from build123d import *

# Parameters (mm, degrees)
F0_R     = 25.4
F0_R_2   = 2.2225
F1_DEPTH = 6.35
F3_R     = 2.54
F2_R     = 2.54
F4_DEPTH = 25.4
F2_R_2   = 7.9375
F5_DEPTH = 25.4
F6_R     = 2.54
F7_DEPTH = 25.4
F8_R     = 2.54
F9_SIZE  = 5.08


with BuildPart() as f1:
    # F0 (on Top) → F1 (new body)
    with BuildSketch(Plane.XY):
        Circle(F0_R)
        with Locations((0, -20.6375)):
            Circle(F0_R_2, mode=Mode.SUBTRACT)
        with Locations((-20.6375, 0)):
            Circle(F0_R_2, mode=Mode.SUBTRACT)
        with Locations((20.6375, 0)):
            Circle(F0_R_2, mode=Mode.SUBTRACT)
        with BuildLine():
            Line((-4.064, 10.31875), (-4.064, 0))
            ThreePointArc((-4.064, 0), (0, -4.064), (4.064, 0))
            Line((4.064, 0), (4.064, 10.31875))
            ThreePointArc((4.064, 10.31875), (7.239, 14.1114143812), (10.414, 10.31875))
            Line((10.414, 10.31875), (10.414, 0))
            ThreePointArc((10.414, 0), (0, -10.414), (-10.414, 0))
            Line((-10.414, 0), (-10.414, 10.31875))
            ThreePointArc((-10.414, 10.31875), (-7.239, 14.1114143812), (-4.064, 10.31875))
        make_face(mode=Mode.SUBTRACT)
        with Locations((0, 20.6375)):
            Circle(F0_R_2, mode=Mode.SUBTRACT)
        with BuildLine():
            ThreePointArc((4.064, 0), (0, -4.064), (-4.064, 0))
            Line((-4.064, 0), (-4.064, 10.31875))
            ThreePointArc((-4.064, 10.31875), (-7.239, 14.1114143812), (-10.414, 10.31875))
            Line((-10.414, 10.31875), (-10.414, 0))
            ThreePointArc((-10.414, 0), (0, -10.414), (10.414, 0))
            Line((10.414, 0), (10.414, 10.31875))
            ThreePointArc((10.414, 10.31875), (7.239, 14.1114143812), (4.064, 10.31875))
            Line((4.064, 10.31875), (4.064, 0))
        make_face()
        with Locations((0, -20.6375)):
            Circle(F0_R_2)
        with Locations((-20.6375, 0)):
            Circle(F0_R_2)
        with Locations((0, 20.6375)):
            Circle(F0_R_2)
        with Locations((20.6375, 0)):
            Circle(F0_R_2)
    extrude(amount=F1_DEPTH)

    # F3
    f3_edges = [f1.edges().sort_by_distance(p)[0] for p in [
        (-25.4, 0, 6.35),
    ]]
    fillet(f3_edges, radius=F3_R)

    # F2 (on face) → F4 (cut)
    with BuildSketch(Plane.XY.offset(6.35)):
        Circle(F2_R)
    extrude(amount=-F4_DEPTH, mode=Mode.SUBTRACT)

    # F2 (on face) → F5 (join)
    with BuildSketch(Plane.XY.offset(6.35)):
        Circle(F2_R_2)
        Circle(F2_R, mode=Mode.SUBTRACT)
    extrude(amount=F5_DEPTH)

    # F6
    f6_edges = [f1.edges().sort_by_distance(p)[0] for p in [
        (-22.86, 0, 6.35),
        (-7.9375, 0, 6.35),
    ]]
    fillet(f6_edges, radius=F6_R)

    # F0 (on Top) → F7 (cut)
    with BuildSketch(Plane.XY):
        with Locations((20.6375, 0)):
            Circle(F0_R_2)
        with Locations((0, 20.6375)):
            Circle(F0_R_2)
        with Locations((-20.6375, 0)):
            Circle(F0_R_2)
        with Locations((0, -20.6375)):
            Circle(F0_R_2)
    extrude(amount=F7_DEPTH, mode=Mode.SUBTRACT)

    # F8
    f8_edges = [f1.edges().sort_by_distance(p)[0] for p in [
        (-7.9375, 0, 31.75),
        (-2.54, 0, 31.75),
    ]]
    fillet(f8_edges, radius=F8_R)

    # F9
    f9_edges = [f1.edges().sort_by_distance(p)[0] for p in [
        (-2.54, 0, 0),
    ]]
    chamfer(f9_edges, length=F9_SIZE)


solid = f1.part
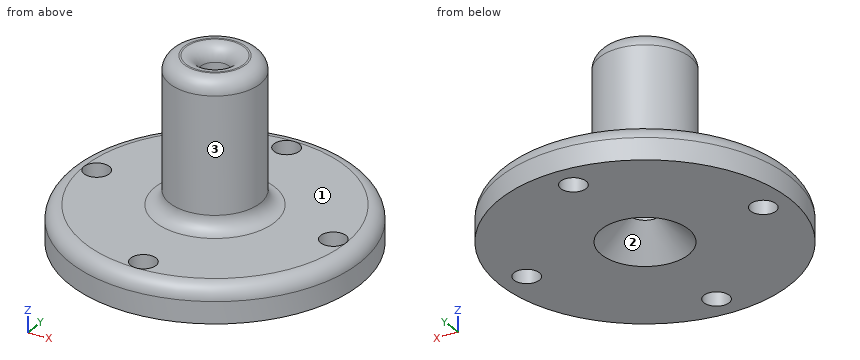
Part model, mm, in its own coordinate system. Face numbers are marked on the shaded views. Coordinates: 2 decimals unless noted, no trailing zeros. Order: outer loops, then holes, each group sorted by start corner. A loop starts at its lowest first (then second) coordinate and runs counter-clockwise, first axis right, second up. Notation, with made-up numbers: (-27.5, 21) - (9.5, 21) arc R20 ccw to (9.5, 30) - close; hole circle Ø7 at (81.25, 19). An arc over 180 degrees is marked (long way). Use CSV: the item, a comma, the result in double quotes.
Item 1: Probe probe 1 along Y at (x, z) = (0, 17.5); probe 2 along Y at (x, z) = (0, 5) (3 decimals); probe 3 along Z at (x, y) = (-3.5, 18). List the from-to ranges inside material, lowest first.
Solved:
probe 1,"y = -7.94 to -2.54, 2.54 to 7.94"
probe 2,"y = -25.104 to -22.86, -18.415 to -2.62, 2.62 to 18.415, 22.86 to 25.104"
probe 3,"z = 0 to 6.35"
Item 2: Mould opens along Y. For the marked faces 1, 2 and 3 say: +Y half, -Y half, draft (parallel to the pull), parting line (faces both ways), or undercut.
Solved:
face 1,"draft"
face 2,"undercut"
face 3,"parting line"
Item 3: Saw through at B-B on z = 30. Give the cut face in (x, y).
Solved:
outline,"circle Ø15.62 at (0, 0); hole circle Ø5.33 at (0, 0)"
Item 4: Drop flat-ended pins along their axis: P1, Ø5, axis at x = -15.5, y = 10, coming from the +Z side; P2, Ø12, axis at y = 9, z = 24, coming from the +X side; P3, Ø5, axis at x = 4, z = 28, coming from the -Y side; P4, Ø23, axis at x = 8, y = -9.5, coming from the +Z side. Give the stop position or say it passes through.
Solved:
P1,"stops at z = 6.35"
P2,"stops at x = 7.35"
P3,"stops at y = -7.79"
P4,"stops at z = 31.75"
Item 5: Saw through at A-A on z = 10. Give the cut face in (x, y) (1 decimal), and give its area (3 significant figures).
Solved:
outline,"circle Ø15.9 at (0, 0); hole circle Ø5.1 at (0, 0)"
area,"178 mm²"
